```python
from build123d import *

# Parameters (mm, degrees)
SKETCH1_W                                  = 92.8
SKETCH1_H                                  = 92.8
BOSS_EXTRUDE1_DEPTH                        = 117
BOSS_EXTRUDE2_START                        = -117
SKETCH2_R                                  = 7.5
BOSS_EXTRUDE2_DEPTH                        = 143.5
BOSS_EXTRUDE3_DEPTH                        = 2
SKETCH4_W                                  = 7.017872994
SKETCH4_H                                  = 7.12386543
BOSS_EXTRUDE4_DEPTH                        = 3
SKETCH5_R                                  = 1
CUT_EXTRUDE1_DEPTH                         = 3.5
CIRPATTERN1_COUNT                          = 4
MIRROR2_AT_THE_SECOND_PLANE_COPY_1_SKETC_R = 1
MIRROR2_AT_THE_SECOND_PLANE_COPY_1_DEPTH   = 3.5


with BuildPart() as part:
    # Sketch1 → Boss-Extrude1 (new body)
    with BuildSketch(Plane(origin=(0, 0, 0), x_dir=(1, 0, 0), z_dir=(0, 1, 0))):
        with Locations((46.4, 46.4)):
            Rectangle(SKETCH1_W, SKETCH1_H)
    extrude(amount=BOSS_EXTRUDE1_DEPTH)

    # Sketch2 → Boss-Extrude2 (add)
    with BuildSketch(Plane(origin=(0, 117, 0), x_dir=(1, 0, 0), z_dir=(0, 1, 0)).offset(BOSS_EXTRUDE2_START)):
        with Locations(Location((46.4, 46.4, 0), (0, 0, 90))):
            Circle(SKETCH2_R)
    extrude(amount=BOSS_EXTRUDE2_DEPTH)

    # Sketch3 → Boss-Extrude3 (add)
    with BuildSketch(Plane(origin=(0, 117, 0), x_dir=(1, 0, 0), z_dir=(0, 1, 0))):
        with BuildLine():
            ThreePointArc((15, 72.8), (18.535533906, 74.264466094), (20, 77.8))
            Line((20, 77.8), (15, 77.8))
            Line((15, 77.8), (15, 72.8))
        make_face()
        with BuildLine():
            Line((15, 77.8), (20, 77.8))
            ThreePointArc((20, 77.8), (11.464466094, 81.335533906), (15, 72.8))
            Line((15, 72.8), (15, 77.8))
        make_face()
        with BuildLine():
            ThreePointArc((15, 72.8), (18.535533906, 74.264466094), (20, 77.8))
            Line((20, 77.8), (15, 77.8))
            Line((15, 77.8), (15, 72.8))
        make_face()
        with BuildLine():
            Line((15, 77.8), (20, 77.8))
            ThreePointArc((20, 77.8), (11.464466094, 81.335533906), (15, 72.8))
            Line((15, 72.8), (15, 77.8))
        make_face()
    boss_extrude3 = extrude(amount=BOSS_EXTRUDE3_DEPTH)

    # Sketch4 → Boss-Extrude4 (add)
    with BuildSketch(Plane(origin=(0, 119, 0), x_dir=(1, 0, 0), z_dir=(0, 1, 0))):
        with Locations((15, 77.8)):
            Rectangle(SKETCH4_W, SKETCH4_H)
    boss_extrude4 = extrude(amount=BOSS_EXTRUDE4_DEPTH)

    # Sketch5 → Cut-Extrude1 (cut)
    with BuildSketch(Plane(origin=(0, 0, -81.361932715), x_dir=(-1, 0, 0), z_dir=(0, 0, -1))):
        with Locations((-15, 120.5)):
            Circle(SKETCH5_R)
    cut_extrude1 = extrude(amount=-CUT_EXTRUDE1_DEPTH, mode=Mode.SUBTRACT)

    # CirPattern1: Boss-Extrude3, Boss-Extrude4 ×4 about axis
    cirpattern1_axis = Axis((46.4, 0, -46.4), (0, 1, 0))
    add([boss_extrude3.rotate(cirpattern1_axis, i * 360 / CIRPATTERN1_COUNT) for i in range(1, CIRPATTERN1_COUNT)])
    add([boss_extrude4.rotate(cirpattern1_axis, i * 360 / CIRPATTERN1_COUNT) for i in range(1, CIRPATTERN1_COUNT)])

    # Mirror1: Cut-Extrude1 across plane
    add(cut_extrude1.mirror(Plane(origin=(0, 0, -46.4), x_dir=(1, 0, 0), z_dir=(0, 0, -1))), mode=Mode.SUBTRACT)

    # Mirror2: Cut-Extrude1 across plane
    add(cut_extrude1.mirror(Plane(origin=(46.4, 0, 0), x_dir=(0, 0, 1), z_dir=(1, 0, 0))), mode=Mode.SUBTRACT)

    # Mirror2 at the second plane: Cut-Extrude1 across plane
    add(cut_extrude1.mirror(Plane(origin=(0, 0, -46.4), x_dir=(1, 0, 0), z_dir=(0, 0, -1))), mode=Mode.SUBTRACT)

    # Mirror2 at the second plane copy 1 sketc → Mirror2 at the second plane copy 1 (cut)
    with BuildSketch(Plane(origin=(92.8, 0, -11.438067285), x_dir=(1, 0, 0), z_dir=(0, 0, 1))):
        with Locations((-15, 120.5)):
            Circle(MIRROR2_AT_THE_SECOND_PLANE_COPY_1_SKETC_R)
    extrude(amount=-MIRROR2_AT_THE_SECOND_PLANE_COPY_1_DEPTH, mode=Mode.SUBTRACT)


solid = part.part
```
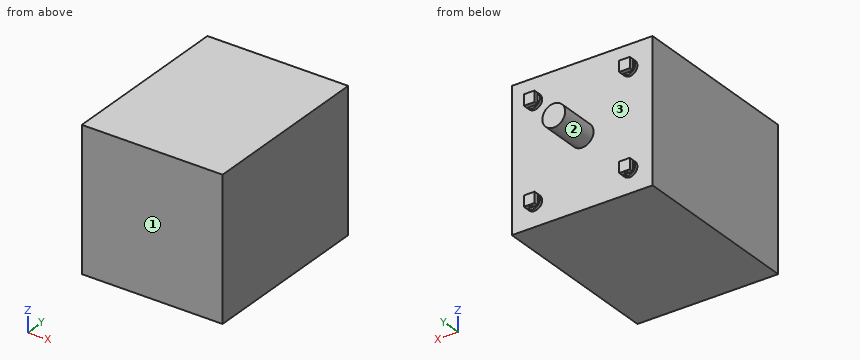
Verification items for the finished model (mm, model axes). Face numbers are marked on the shaded views. Coordinates: 2 decimals unless noted, no trailing zeros. Order: outer loops, then holes, each group sorted by start corner. A loop starts at its lowest first (then second) coordinate and runs counter-clockwise, first axis right, second up. Notation, with made-up numbers: (64.25, -32) -> (83.25, -32) arc R21 ccw to (83.25, 2) -> close; hole circle Ø6 at (48.25, -19.75). An arc over 180 degrees is marked (long way). Put each result on its own line as item: value. Start each with the question number.
1) Cross-section at D-D (x = 87). Enter the section's corners in (y, z).
2) Release check for a two-part mould opening along Z. For the marked faces 1, 2 and 3 record: pulls with the +Z half, pulls with the -Z half, needs draft (parallel to the pull), parting line crosses it, or undercut.
3) Cross-section at B-B (x = 46.4). Enter the section's corners in (y, z), plus the area to 3 significant figures.
4) Cross-section at C-C (z = -22.5). Enter the section's corners in (x, y).
5) Go/stop test with flat-tipped pins: pin 1 (2 mm diameter, centred on x = 73, z = -49, fed in from +Y); pin 2 (10 mm diameter, centred on x = 73.5, z = -69.5, fed in from +Y); pin 3 (0.9 mm diameter, centred on x = 79.5, y = 120, fed in from +Z). Record where each tip stops, or that it passes through.
6) Cross-section at A-A (z = -46.4). Enter the section's corners in (x, y).
7) Material ranges on L1, parallel to X at y = 120.5, z = -79.35; L2, parallel to X at y = 120.5, z = -13.7; L3, parallel to Y at x = 56, z = -39, recorded low to high.
Geometry check:
1. outline: (0, -92.8) -> (117, -92.8) -> (117, 0) -> (0, 0) -> close
2. face 1: needs draft
2. face 2: parting line crosses it
2. face 3: undercut
3. outline: (0, -92.8) -> (117, -92.8) -> (117, -53.9) -> (143.5, -53.9) -> (143.5, -38.9) -> (117, -38.9) -> (117, 0) -> (0, 0) -> close
3. area: 11,300 mm^2
4. outline: (0, 0) -> (92.8, 0) -> (92.8, 117) -> (0, 117) -> close
5. pin 1: stops at y = 117
5. pin 2: stops at y = 122
5. pin 3: stops at z = -11.44
6. outline: (0, 0) -> (92.8, 0) -> (92.8, 117) -> (53.9, 117) -> (53.9, 143.5) -> (38.9, 143.5) -> (38.9, 117) -> (0, 117) -> close
7. L1: x = 11.49 to 14, 16 to 18.51, 74.24 to 76.8, 78.8 to 81.36
7. L2: x = 11.44 to 14, 16 to 18.56, 74.29 to 76.8, 78.8 to 81.31
7. L3: y = 0 to 117
